from build123d import *

# Parameters (mm, degrees)
SKETCH1_R           = 9.09
BOSS_EXTRUDE1_DEPTH = 13.52
SKETCH2_R           = 5.885
BOSS_EXTRUDE2_DEPTH = 9.41
SKETCH3_OUTSIDE_W   = 27.07
SKETCH3_OUTSIDE_H   = 27.07
SKETCH3_OUTSIDE_R   = 7.78
CUT_EXTRUDE1_DEPTH  = 12.32
SKETCH4_R           = 9.09
BOSS_EXTRUDE3_DEPTH = 1.2
SKETCH5_R           = 2.5
CUT_EXTRUDE2_DEPTH  = 23.93
FILLET3_R           = 0.3


with BuildPart() as part:
    # Sketch1 → Boss-Extrude1 (new body)
    with BuildSketch(Plane(origin=(0, 0, 0), x_dir=(1, 0, 0), z_dir=(0, 1, 0))):
        Circle(SKETCH1_R)
    extrude(amount=BOSS_EXTRUDE1_DEPTH)

    # Sketch2 → Boss-Extrude2 (add)
    with BuildSketch(Plane(origin=(0, 13.52, 0), x_dir=(1, 0, 0), z_dir=(0, 1, 0))):
        Circle(SKETCH2_R)
    extrude(amount=BOSS_EXTRUDE2_DEPTH)

    # Sketch3 outside → Cut-Extrude1 (cut)
    with BuildSketch(Plane.XZ):
        Rectangle(SKETCH3_OUTSIDE_W, SKETCH3_OUTSIDE_H)
        Circle(SKETCH3_OUTSIDE_R, mode=Mode.SUBTRACT)
    extrude(amount=-CUT_EXTRUDE1_DEPTH, mode=Mode.SUBTRACT)

    # Sketch4 → Boss-Extrude3 (add)
    with BuildSketch(Plane.XZ):
        Circle(SKETCH4_R)
    extrude(amount=-BOSS_EXTRUDE3_DEPTH)

    # Sketch5 → Cut-Extrude2 (cut, through all)
    with BuildSketch(Plane.XZ):
        Circle(SKETCH5_R)
    extrude(amount=-CUT_EXTRUDE2_DEPTH, mode=Mode.SUBTRACT)

    # Fillet3
    fillet3_edges = [part.edges().sort_by_distance(p)[0] for p in [
        (-2.5, 22.93, 0),
        (-2.5, 0, 0),
        (-5.885, 22.93, 0),
    ]]
    fillet(fillet3_edges, radius=FILLET3_R)


solid = part.part
Can you work these out from the model? Positions are in its coordinate system, mm. A direction names the side the tool comes from. Round coordinates to 2 decimals unless told otherwise and drop trailing zeros. Order: outer loops, then holes, each group sorted by start corner. A loop starts at its lowest first (then second) coordinate and runs counter-clockwise, first axis right, second up. Notation, with made-up numbers: (28.25, -3) -> (46.25, -3) arc R21 cw to (46.25, 18) -> close; hole circle Ø3 at (-4, 80). An arc over 180 degrees is marked (long way). Write each question's results on one line, items separated by ' | '. Start each with the question number.
Item 1: Please list where these lines run through material, in increasing order: L1, parallel to Z at x = 0, y = 6.5; L2, parallel to Z at x = 0, y = 15 (3 decimals); L3, parallel to Y at x = -6.75, z = 4.25.
Item 2: If we section it at D-D, the plane y = 18.75: Write out the boundary of the cut face in (x, z) (3 decimals), then the cut area to 3 significant figures.
Item 3: If we section it at C-C, the plane y = 6.25: Write out the boundary of the cut face in (x, z).
Item 4: If we section it at A-A, the plane z = 0: Write out the boundary of the cut face in (x, y) (3 decimals).
Item 5: Which directions (+Z, -Z, +X, -X, +Y, -Y) give clear straight access to the entire face, cutting with the end or side of a thin tool? Please do faces 4 (the cylindrical face through (-6.7, 12.912, -6.143)), 5 (the flat face through (7, 1.2, 4)), 6 (the cylindrical face through (-5.88, 18.01, -0.26)).
Item 6: Thinking about a two-plate mould opening in X: for faces 1 (the flat face through (2, 13.52, 6)), 2 (the cylindrical face through (-6.7, 0.592, 6.143)), 3 (the cylindrical face through (-0.54, 11.31, -2.44)), which applies, +X half, -X half, draft (parallel to the pull), parting line (faces both ways), or undercut?
Item 7: If we section it at B-B, the plane x = 0: Write out the boundary of the cut face in (y, z) (3 decimals), then the cut area to 3 significant figures.
Item 8: Will these pins go through, and if not, where does the flat tip stop? pin 1 (1.5 mm diameter, centred on x = 1, z = -0.5, fed in from -Y); pin 2 (1 mm diameter, centred on x = 0.5, y = 6, fed in from +Z); pin 3 (1 mm diameter, centred on x = 5, z = 7, fed in from +Y); pin 4 (2 mm diameter, centred on y = 4, z = 0.5, fed in from -X).
Results:
1) L1: z = -7.78 to -2.5, 2.5 to 7.78 | L2: z = -5.885 to -2.5, 2.5 to 5.885 | L3: y = 0 to 1.2, 12.32 to 13.52
2) outline: circle Ø11.77 at (0, 0); hole circle Ø5 at (0, 0) | area: 89.2 mm2
3) outline: circle Ø15.56 at (0, 0); hole circle Ø5 at (0, 0)
4) outline: (-9.09, 0) -> (-2.8, 0) arc R0.3 ccw to (-2.5, 0.3) -> (-2.5, 22.63) arc R0.3 ccw to (-2.8, 22.93) -> (-5.585, 22.93) arc R0.3 ccw to (-5.885, 22.63) -> (-5.885, 13.52) -> (-9.09, 13.52) -> (-9.09, 12.32) -> (-7.78, 12.32) -> (-7.78, 1.2) -> (-9.09, 1.2) -> close; (2.5, 0.3) arc R0.3 ccw to (2.8, 0) -> (9.09, 0) -> (9.09, 1.2) -> (7.78, 1.2) -> (7.78, 12.32) -> (9.09, 12.32) -> (9.09, 13.52) -> (5.885, 13.52) -> (5.885, 22.63) arc R0.3 ccw to (5.585, 22.93) -> (2.8, 22.93) arc R0.3 ccw to (2.5, 22.63) -> close
5) face 4: +Y, -Y | face 5: none | face 6: +Y
6) face 1: draft | face 2: parting line | face 3: undercut
7) outline: (0, -9.09) -> (1.2, -9.09) -> (1.2, -7.78) -> (12.32, -7.78) -> (12.32, -9.09) -> (13.52, -9.09) -> (13.52, -5.885) -> (22.63, -5.885) arc R0.3 ccw to (22.93, -5.585) -> (22.93, -2.8) arc R0.3 ccw to (22.63, -2.5) -> (0.3, -2.5) arc R0.3 ccw to (0, -2.8) -> close; (0, 2.8) arc R0.3 ccw to (0.3, 2.5) -> (22.63, 2.5) arc R0.3 ccw to (22.93, 2.8) -> (22.93, 5.585) arc R0.3 ccw to (22.63, 5.885) -> (13.52, 5.885) -> (13.52, 9.09) -> (12.32, 9.09) -> (12.32, 7.78) -> (1.2, 7.78) -> (1.2, 9.09) -> (0, 9.09) -> close | area: 213 mm2
8) pin 1: passes through | pin 2: stops at z = 7.78 | pin 3: stops at y = 13.52 | pin 4: stops at x = -7.78
